Build history of the part. All positions in model axes, mm. A direction names the side the tool comes from. Coordinates: 2 decimals unless noted, no trailing zeros. Write each loop counter-clockwise with the first axis right and the second up, starting at its lowest first coordinate (ties: lowest second). Pieces come first, ordered by that corner, then holes.
from build123d import *

# Parameters (mm, degrees)
F1_DEPTH = 10
F2_W     = 6
F2_H     = 6
F2_W_2   = 8
F2_H_2   = 8
F3_DEPTH = 2
F4_DEPTH = 10


with BuildPart() as f1:
    # F0 (on Top) → F1 (new body)
    with BuildSketch(Plane.XY):
        Polygon((-0.5, 0.5), (-1.5, 0.5), (-1.5, -0.5), (-0.5, -0.5), (-0.5, -1.5), (0.5, -1.5), (0.5, -0.5), (1.5, -0.5), (1.5, 0.5), (0.5, 0.5), (0.5, 1.5), (-0.5, 1.5), align=None)
    extrude(amount=F1_DEPTH)

    # F2 (on face) → F3 (join)
    with BuildSketch(Plane.XY.offset(10)):
        Rectangle(F2_W_2, F2_H_2)
        Rectangle(F2_W, F2_H, mode=Mode.SUBTRACT)
        Rectangle(F2_W, F2_H)
        Polygon((-1.5, 0.5), (-0.5, 0.5), (-0.5, 1.5), (0.5, 1.5), (0.5, 0.5), (1.5, 0.5), (1.5, -0.5), (0.5, -0.5), (0.5, -1.5), (-0.5, -1.5), (-0.5, -0.5), (-1.5, -0.5), align=None, mode=Mode.SUBTRACT)
    extrude(amount=-F3_DEPTH)

    # F2 (on face) → F4 (join)
    with BuildSketch(Plane.XY.offset(10)):
        Rectangle(F2_W_2, F2_H_2)
        Rectangle(F2_W, F2_H, mode=Mode.SUBTRACT)
    extrude(amount=F4_DEPTH)


solid = f1.part
(1) Slice it at A-A, the plane z = 16.5. List the corners of the cut face in (x, y).
(2) Probe L1, parallel to X at y = 1.5, z = 13.5; L2, parallel to Z at x = -1, y = 3.25. List the from-to ranges inside material, lowest first.
(3) Slice it at C-C, the plane x = -1.75. List the corners of the cut face in (y, z).
(4) 3-axis set-ups, long thin cutter, end or side, ignore diameter. For faces 5 (the flat face through (1, 0.5, 4)), 6 (the flat face through (0.5, -1, 4)), 7 (the flat face through (0, -1.5, 4)), 8 (the flat face through (0, -3, 15)), 9 (the flat face through (1.5, 0, 4)): which of +Z, -Z, +X, -X, +Y, -Y reach the whole face in a straight line?
(5) Slice it at D-D, the plane z = 4.25. List the corners of the cut face in (x, y).
(6) Flat gauge pins, fed straight in: P1, Ø0.5, axis at x = 0, z = 4, coming from the +Y side; P2, Ø1.1, axis at y = 0, z = 4, coming from the +X side; P3, Ø0.8, axis at x = -1, z = 5.5, coming from the -Y side. Where does each tip first touch, or does it go through?
(7) Slice it at B-B, the plane y = 0. List the corners of the cut face in (x, z), and give its area (3 significant figures).
(8) Two-plate mould, pull along Y, no slides. Class faces 1 (the flat face through (-1.5, 0, 4)), 2 (the flat face through (1, -0.5, 4)), 3 (the flat face through (0, 0, 10)), 4 (the flat face through (0, 1.5, 4)): pulls with the +Y half, pulls with the -Y half, needs draft (parallel to the pull), parting line crosses it, or undercut.
Results:
1. outline: (-4, -4) - (4, -4) - (4, 4) - (-4, 4) - close; hole (-3, -3) - (3, -3) - (3, 3) - (-3, 3) - close
2. L1: x = -4 to -3, 3 to 4
2. L2: z = 8 to 20
3. outline: (-4, 8) - (4, 8) - (4, 20) - (3, 20) - (3, 10) - (-3, 10) - (-3, 20) - (-4, 20) - close
4. face 5: -Z, +X, +Y
4. face 6: -Z, +X, -Y
4. face 7: -Z, +X, -X, -Y
4. face 8: +Z
4. face 9: -Z, +X, +Y, -Y
5. outline: (-1.5, -0.5) - (-0.5, -0.5) - (-0.5, -1.5) - (0.5, -1.5) - (0.5, -0.5) - (1.5, -0.5) - (1.5, 0.5) - (0.5, 0.5) - (0.5, 1.5) - (-0.5, 1.5) - (-0.5, 0.5) - (-1.5, 0.5) - close
6. P1: stops at y = 1.5
6. P2: stops at x = 1.5
6. P3: stops at y = -0.5
7. outline: (-4, 8) - (-1.5, 8) - (-1.5, 0) - (1.5, 0) - (1.5, 8) - (4, 8) - (4, 20) - (3, 20) - (3, 10) - (-3, 10) - (-3, 20) - (-4, 20) - close
7. area: 60.0 mm2
8. face 1: needs draft
8. face 2: pulls with the -Y half
8. face 3: undercut
8. face 4: pulls with the +Y half
